from build123d import *

# Parameters (mm, degrees)
SKETCH1_W            = 200
SKETCH1_H            = 120
SKETCH1_W_2          = 160
SKETCH1_H_2          = 80
BOSS_EXTRUDE1_DEPTH  = 1
FILLET1_R            = 2
M5_CLEARANCE_HOLE1_D = 5.8


with BuildPart() as part:
    # Sketch1 → Boss-Extrude1 (new body)
    with BuildSketch(Plane.XY):
        Rectangle(SKETCH1_W, SKETCH1_H)
        Rectangle(SKETCH1_W_2, SKETCH1_H_2, mode=Mode.SUBTRACT)
    extrude(amount=BOSS_EXTRUDE1_DEPTH)

    # Fillet1
    fillet1_edges = [part.edges().sort_by_distance(p)[0] for p in [
        (-80, 40, 0.5),
        (-80, -40, 0.5),
        (80, -40, 0.5),
        (80, 40, 0.5),
        (-100, 60, 0.5),
        (100, 60, 0.5),
        (100, -60, 0.5),
        (-100, -60, 0.5),
    ]]
    fillet(fillet1_edges, radius=FILLET1_R)

    # M5 Clearance Hole1 (through all)
    with Locations(Plane.XY.offset(1)):
        with Locations((92, -30.334149623), (69.646446609, -52.66277265), (92, 30.107073019), (0, -52.66277265), (69.646446609, 52.435696047), (0, 52.435696047), (-69.646446609, 52.435696047), (-92, 30.107073019), (-92, -30.334149623), (-69.646446609, -52.66277265)):
            Hole(M5_CLEARANCE_HOLE1_D / 2)


solid = part.part
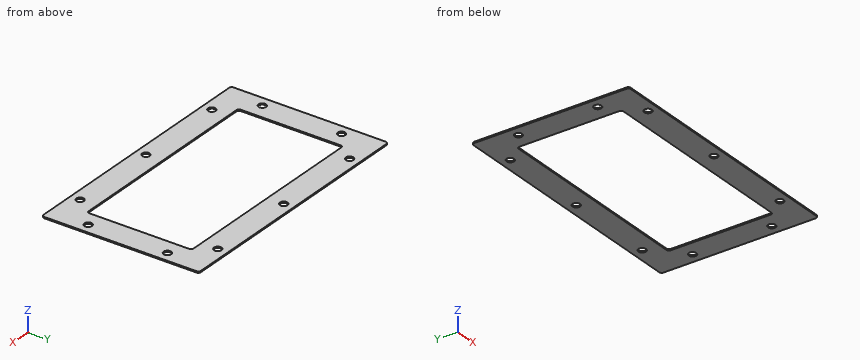
Could you check a few things on this model? Use its own coordinates, in mm. Round coordinates to 2 decimals unless told otherwise and drop trailing zeros. Write each loop counter-clockwise with the first axis right and the second up, starting at its lowest first coordinate (ties: lowest second). Pieces come first, ordered by that corner, then holes. Notation, with made-up numbers: (61.25, -6) - (87.25, -6) arc R13 cw to (87.25, -2) - close; hole circle Ø5 at (-27, 52.25). An arc over 180 degrees is marked (long way). Put each result on its own line as item: value. Start each with the question number.
(1) Will this pin go through, and if not, where does the flat tip stop? pin 1 (4.5 mm diameter, centred on x = 92, y = -30.33, fed in from -Z).
(2) I need wall thicknesses on probe 1 along Y at (x, z) = (0, 0.5); probe 2 along Y at (x, z) = (92, 0.85); probe 3 along Y at (x, z) = (74, 0.55). Which ranges of each line are inside material? Lowest first, please.
(3) I want a section at D-D, the plane x = 92. Please give me the cut outline in (y, z).
(4) I want a section at C-C, the plane x = -26.5. Please give me the cut outline in (y, z).
(5) I want a section at B-B, the plane y = 35. Please give me the cut outline in (x, z).
(6) I want a section at A-A, the plane x = 0. Please give me the cut outline in (y, z), plus the area to 3 significant figures.
Here are the results:
1. pin 1: passes through
2. probe 1: y = -60 to -55.56, -49.76 to -40, 40 to 49.54, 55.34 to 60
2. probe 2: y = -60 to -33.23, -27.43 to 27.21, 33.01 to 60
2. probe 3: y = -60 to -40, 40 to 60
3. outline: (-60, 0) - (-33.23, 0) - (-33.23, 1) - (-60, 1) - close; (-27.43, 0) - (27.21, 0) - (27.21, 1) - (-27.43, 1) - close; (33.01, 0) - (60, 0) - (60, 1) - (33.01, 1) - close
4. outline: (-60, 0) - (-40, 0) - (-40, 1) - (-60, 1) - close; (40, 0) - (60, 0) - (60, 1) - (40, 1) - close
5. outline: (-100, 0) - (-80, 0) - (-80, 1) - (-100, 1) - close; (80, 0) - (100, 0) - (100, 1) - (80, 1) - close
6. outline: (-60, 0) - (-55.56, 0) - (-55.56, 1) - (-60, 1) - close; (-49.76, 0) - (-40, 0) - (-40, 1) - (-49.76, 1) - close; (40, 0) - (49.54, 0) - (49.54, 1) - (40, 1) - close; (55.34, 0) - (60, 0) - (60, 1) - (55.34, 1) - close
6. area: 28.4 mm^2
